from build123d import *

# Parameters (mm, degrees)
BOSS_EXTRUDE1_DEPTH = 19.05


with BuildPart() as part:
    # Sketch1 → Boss-Extrude1 (new body)
    with BuildSketch(Plane(origin=(0, 0, 0), x_dir=(1, 0, 0), z_dir=(0, 1, 0))):
        with BuildLine():
            Line((50.8, -279.4), (0, -279.4))
            Line((0, -279.4), (0, 0))
            Line((0, 0), (52.907108287, 0))
            ThreePointArc((52.907108287, 0), (22.753262856, -58.398850563), (23.389451167, -124.120045058))
            Line((23.389451167, -124.120045058), (60.329571515, -267.095372264))
            ThreePointArc((60.329571515, -267.095372264), (58.58165466, -275.584162178), (50.8, -279.4))
        make_face()
    extrude(amount=BOSS_EXTRUDE1_DEPTH)


solid = part.part
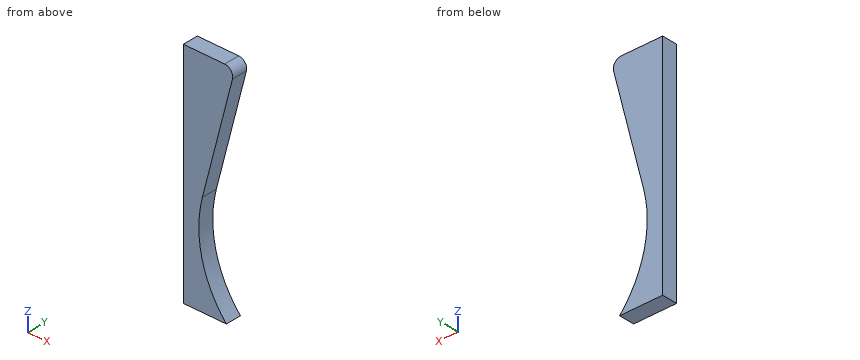
Source: CAD feature listing. Evaluate the final solid. Frame: model axes, mm. Coordinates: 2 decimals unless noted, no trailing zeros. Loops run counter-clockwise (first coordinate to the right, second up) from the corner with the lowest first, then second, coordinate; pieces in that order, holes last. Notation, with made-up numbers: (-17, -35.75) - (-4, -35.75) arc R28 ccw to (-4, -17.75) - close; hole circle Ø11 at (28, 5). An arc over 180 degrees is marked (long way). One line per item, written item: value. Start each with the question number.
1. Section B-B (y = 14.25). Return the cut outline in (x, z) (1 decimal).
2. Ray query, L1, parallel to X at y = 17, z = 112.5; L2, parallel to X at y = 1.5, z = 55. Return the intervals inside material, ascending.
3. Section A-A (x = 26.5). Return the cut outline in (y, z), and give its area (3 significant figures).
4. Section D-D (x = 44.5). Return the cut outline in (y, z).
5. Contact query for flat-ended pins moving along their axis: P1, Ø12, axis at x = 10, z = 32, coming from the -Y side; P2, Ø1, axis at y = 10.5, z = 157.5, coming from the +X side; P3, Ø8, axis at y = 12.5, z = 167.5, coming from the +X side; P4, Ø4, axis at y = 5.5, z = 114, coming from the +X side. Output: stop coordinate, or through.
6. Section C-C (z = 185.5). Return the cut outline in (x, y).
Verdict:
1. outline: (0, 0) - (52.9, 0) arc R136.5 cw to (23.4, 124.1) - (60.3, 267.1) arc R9.8 ccw to (50.8, 279.4) - (0, 279.4) - close
2. L1: x = 0 to 20.92
2. L2: x = 0 to 23.61
3. outline: (0, 0) - (19.05, 0) - (19.05, 45.5) - (0, 45.5) - close; (0, 136.16) - (19.05, 136.16) - (19.05, 279.4) - (0, 279.4) - close
3. area: 3,600 mm2
4. outline: (0, 0) - (19.05, 0) - (19.05, 10.61) - (0, 10.61) - close; (0, 205.83) - (19.05, 205.83) - (19.05, 279.4) - (0, 279.4) - close
5. P1: stops at y = 0
5. P2: stops at x = 32.14
5. P3: stops at x = 35.63
5. P4: stops at x = 21.55
6. outline: (0, 0) - (39.25, 0) - (39.25, 19.05) - (0, 19.05) - close
